from build123d import *

# Parameters (mm, degrees)
BOSS_EXTRUDE1_DEPTH = 3
FILLET2_R           = 10
FILLET1_R           = 1.5


with BuildPart() as part:
    # Sketch1 → Boss-Extrude1 (new body)
    with BuildSketch(Plane(origin=(0, 0, 0), x_dir=(1, 0, 0), z_dir=(0, 1, 0))):
        Polygon((0, 0), (120, 0), (120, 70), (80, 60), align=None)
    extrude(amount=BOSS_EXTRUDE1_DEPTH)

    # Fillet2
    fillet2_edges = [part.edges().sort_by_distance(p)[0] for p in [
        (80, 1.5, -60),
    ]]
    fillet(fillet2_edges, radius=FILLET2_R)

    # Fillet1
    fillet1_edges = [part.edges().sort_by_distance(p)[0] for p in [
        (120, 3, -35),
        (120, 0, -35),
        (100.979557811, 3, -65.244889453),
        (100.979557811, 0, -65.244889453),
        (39.192235936, 0, -29.394176952),
        (39.192235936, 3, -29.394176952),
        (80.086755182, 0, -59.817729921),
        (80.086755182, 3, -59.817729921),
    ]]
    fillet(fillet1_edges, radius=FILLET1_R - 0.0001)  # a hair under: the kernel refuses the full size


solid = part.part
Can you work these out from the model? Positions are in its coordinate system, mm. Give positions to 0.01 mm unless a question says otherwise; leave off trailing zeros. Order: outer loops, then holes, each group sorted by start corner. A loop starts at its lowest first (then second) coordinate and runs counter-clockwise, first axis right, second up. Notation, with made-up numbers: M 28,-39 L 63,-39 A23 cw 63,-31 Z; hole C 32,-8.75 d6. An arc over 180 degrees is marked long. Use one line per item in the form item = value.
Item 1: If I drill on line 1 along X through (y, z) = (1.75, -58); line 2 along X through (y, z) = (2.3, -28.5); line 3 along Z through (x, y) = (33, 2.05), over which ranges is the centre line in solid material (lowest first)? Write a range as [from, to].
Values follow:
line_1 = [77.37, 119.98]
line_2 = [38.39, 119.77]
line_3 = [-24.62, 0]
Item 2: If we section it at A-A, the plane y = 0.8: Write out the boundary of the cut face in (x, z).
Values follow:
outline = M 0.29,0 L 78.49,-58.65 A9.83 ccw 82,-60.32 L 119.83,-69.78 L 119.83,0 Z
Item 3: Will these pins go through, and if not, where does the flat tip stop? pin 1 Ø1 at (y, z) = (1, -18) entering from -X; pin 2 Ø5 at (x, z) = (29, -24) entering from +Y.
Values follow:
pin_1 = 23.43
pin_2 = 2.77
